Design review of the part built by this model. Coordinates are the model's own, in mm. A direction names the side the tool comes from. Coordinates: 2 decimals unless noted, no trailing zeros. Order: outer loops, then holes, each group sorted by start corner. A loop starts at its lowest first (then second) coordinate and runs counter-clockwise, first axis right, second up. Notation, with made-up numbers: (-8, -5) -> (16, -5) arc R21 cw to (16, 17) -> close; hole circle Ø6 at (-31, -15). An arc over 180 degrees is marked (long way). Write item = value, one per line.
```python
from build123d import *

# Parameters (mm, degrees)
SKETCH_1_R      = 6
SKETCH_1_R_2    = 24
EXTRUDE_1_DEPTH = 10


with BuildPart() as part:
    # Эскиз1 → Бобышка-Вытянуть1 (new body)
    with BuildSketch(Plane.XY):
        with BuildLine():
            ThreePointArc((-41, 50), (-27.709365364, 48.201234745), (-15.375, 42.934361239))
            ThreePointArc((-15.375, 42.934361239), (0, 38.694977982), (15.375, 42.934361239))
            ThreePointArc((15.375, 42.934361239), (27.709365364, 48.201234745), (41, 50))
            ThreePointArc((41, 50), (47.941363325, 47.78864011), (52.324417909, 41.969579199))
            ThreePointArc((52.324417909, 41.969579199), (64.154153471, 23.154153471), (82.969579199, 11.324417909))
            ThreePointArc((82.969579199, 11.324417909), (91, 0), (82.969579199, -11.324417909))
            ThreePointArc((82.969579199, -11.324417909), (64.154153471, -23.154153471), (52.324417909, -41.969579199))
            ThreePointArc((52.324417909, -41.969579199), (47.941363325, -47.78864011), (41, -50))
            ThreePointArc((41, -50), (27.709365364, -48.201234745), (15.375, -42.934361239))
            ThreePointArc((15.375, -42.934361239), (0, -38.694977982), (-15.375, -42.934361239))
            ThreePointArc((-15.375, -42.934361239), (-27.709365364, -48.201234745), (-41, -50))
            ThreePointArc((-41, -50), (-47.941363325, -47.78864011), (-52.324417909, -41.969579199))
            ThreePointArc((-52.324417909, -41.969579199), (-64.154153471, -23.154153471), (-82.969579199, -11.324417909))
            ThreePointArc((-82.969579199, -11.324417909), (-91, 0), (-82.969579199, 11.324417909))
            ThreePointArc((-82.969579199, 11.324417909), (-64.154153471, 23.154153471), (-52.324417909, 41.969579199))
            ThreePointArc((-52.324417909, 41.969579199), (-47.941363325, 47.78864011), (-41, 50))
        make_face()
        with Locations((-79, 0)):
            Circle(SKETCH_1_R, mode=Mode.SUBTRACT)
        with Locations((-41, 0)):
            Circle(SKETCH_1_R_2, mode=Mode.SUBTRACT)
        with Locations((41, 0)):
            Circle(SKETCH_1_R_2, mode=Mode.SUBTRACT)
        with Locations((79, 0)):
            Circle(SKETCH_1_R, mode=Mode.SUBTRACT)
        with Locations((41, -38)):
            Circle(SKETCH_1_R, mode=Mode.SUBTRACT)
        with Locations((41, 38)):
            Circle(SKETCH_1_R, mode=Mode.SUBTRACT)
        with Locations((0, 25.5)):
            Circle(SKETCH_1_R, mode=Mode.SUBTRACT)
        with Locations((0, -25.5)):
            Circle(SKETCH_1_R, mode=Mode.SUBTRACT)
        with Locations((-41, -38)):
            Circle(SKETCH_1_R, mode=Mode.SUBTRACT)
        with Locations((-41, 38)):
            Circle(SKETCH_1_R, mode=Mode.SUBTRACT)
    extrude(amount=EXTRUDE_1_DEPTH)


solid = part.part
```
(1) The part is to be moulded in two halves that separate along Y. For faces 3 (the cylindrical face through (-18.11, 7.21, 4.93)), 4 (the cylindrical face through (36.24, -41.65, 4.93)), 5 (the cylindrical face through (-48.026, 47.728, 4.93)), 6 (the cylindrical face through (64.38, -22.93, 4.93)), say which applies: released by +Y, released by -Y, zero draft, split by the parting line, or undercut.
Report:
face_3 = undercut
face_4 = undercut
face_5 = released by +Y
face_6 = released by -Y
(2) For faces 1 (the flat face through (0, -3, 10)), 2 (the cylindrical face through (-27.53, -48.15, 4.93)), list the 3-axis set-ups (+Z, -Z, +X, -X, +Y, -Y) from which the entire face can be reached by the end or side of a thin tool; tool diameter is ignored.
Report:
face_1 = +Z, +X, -X, +Y, -Y
face_2 = +Z, -Z, -Y
(3) Insertion check: pin 1 (14 mm diameter, centred on x = 41, y = -38, fed in from +Z); pin 2 (2 mm diameter, centred on x = 51.5, z = 7.5, fed in from +Y); pin 3 (1.5 mm diameter, centred on x = 46, z = 7, fed in from +Y); pin 4 (6 mm diameter, centred on y = 30, z = 5.5, fed in from +X). Each pin has a flat end and moves straight along its axis. Give the tip position at first contact, or say it passes through.
Report:
pin_1 = 10
pin_2 = 45.33
pin_3 = 49.22
pin_4 = 60.69
(4) We need section C-C (y = -16.5). Write out the cut boundary in (x, z), and give its area (3 significant figures).
Report:
outline = (-72.39, 0) -> (-58.43, 0) -> (-58.43, 10) -> (-72.39, 10) -> close; (-23.57, 0) -> (23.57, 0) -> (23.57, 10) -> (-23.57, 10) -> close; (58.43, 0) -> (72.39, 0) -> (72.39, 10) -> (58.43, 10) -> close
area = 751 mm²
(5) We need section A-A (z = 6.5). Give the number of separate pieces and of enclosed holes in the cut face, and give its area (3 significant figures).
Report:
separate_pieces = 1
enclosed_holes = 10
area = 7,950 mm²
(6) For L1, parallel to Y at x = 41, z = 3.75; L2, parallel to X at y = -1, z = 1.25; L3, parallel to X at y = 0.5, z = 7, list the stretches that pass through material, from the lowest coordinate up.
Report:
L1 = -50 to -44, -32 to -24, 24 to 32, 44 to 50
L2 = -90.96 to -84.92, -73.08 to -64.98, -17.02 to 17.02, 64.98 to 73.08, 84.92 to 90.96
L3 = -90.99 to -84.98, -73.02 to -64.99, -17.01 to 17.01, 64.99 to 73.02, 84.98 to 90.99
(7) We need section D-D (x = -79). Write out the cut boundary in (y, z), and give its area (3 significant figures).
Report:
outline = (-12.91, 0) -> (-6, 0) -> (-6, 10) -> (-12.91, 10) -> close; (6, 0) -> (12.91, 0) -> (12.91, 10) -> (6, 10) -> close
area = 138 mm²
(8) We need section B-B (y = 0). Write out the cut boundary in (x, z), and give its area (3 significant figures).
Report:
outline = (-91, 0) -> (-85, 0) -> (-85, 10) -> (-91, 10) -> close; (-73, 0) -> (-65, 0) -> (-65, 10) -> (-73, 10) -> close; (-17, 0) -> (17, 0) -> (17, 10) -> (-17, 10) -> close; (65, 0) -> (73, 0) -> (73, 10) -> (65, 10) -> close; (85, 0) -> (91, 0) -> (91, 10) -> (85, 10) -> close
area = 620 mm²
